Here's how the part is built. I have some questions about the finished solid (model axes, mm). Face numbers are marked on the shaded views. A direction names the side the tool comes from. Round coordinates to 2 decimals unless told otherwise and drop trailing zeros. Loops run counter-clockwise (first coordinate to the right, second up) from the corner with the lowest first, then second, coordinate; pieces in that order, holes last. Notation, with made-up numbers: M 28,65 L 68,65 A20 cw 68,92 Z; hole C 9,-16 d11. An arc over 180 degrees is marked long. Use a Markdown table: item, result.
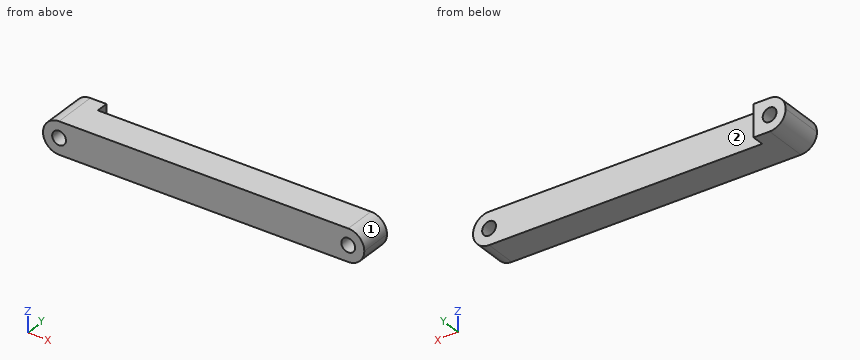
```python
from build123d import *

# Parameters (mm, degrees)
SKETCH_1_W          = 100
SKETCH_1_H          = 10
EXTRUDE_1_DEPTH     = 10
SKETCH_4_W          = 10
SKETCH_4_H          = 10
EXTRUDE_2_DEPTH     = 3.8
FILLET_1_R          = 5
SKETCH_2_R          = 2.15
CUT_EXTRUDE_1_DEPTH = 53.824615474


with BuildPart() as part:
    # 스케치1 → 보스-돌출1 (new body)
    with BuildSketch(Plane.XY):
        Rectangle(SKETCH_1_W, SKETCH_1_H)
    extrude(amount=EXTRUDE_1_DEPTH)

    # 스케치4 → 보스-돌출2 (add)
    with BuildSketch(Plane(origin=(0, 5, 0), x_dir=(1, 0, 0), z_dir=(0, 1, 0))):
        with Locations((-45, -5)):
            Rectangle(SKETCH_4_W, SKETCH_4_H)
    extrude(amount=EXTRUDE_2_DEPTH)

    # 필렛1
    fillet_1_edges = [part.edges().sort_by_distance(p)[0] for p in [
        (50, 0, 0),
        (50, 0, 10),
        (-50, 1.9, 0),
        (-50, 1.9, 10),
    ]]
    fillet(fillet_1_edges, radius=FILLET_1_R - 0.0001)  # a hair under: the kernel refuses the full size

    # 스케치2 → 컷-돌출1 (cut, through all)
    with BuildSketch(Plane(origin=(0, 8.8, 0), x_dir=(1, 0, 0), z_dir=(0, 1, 0))):
        with Locations(Location((-45, -5, 0), (0, 0, 270))):
            Circle(SKETCH_2_R)
        with Locations(Location((45, -5, 0), (0, 0, 270))):
            Circle(SKETCH_2_R)
    extrude(amount=-CUT_EXTRUDE_1_DEPTH, mode=Mode.SUBTRACT)


solid = part.part
```
Q1. For the marked faces 1 and 2, which set-ups out of +Z, -Z, +X, -X, +Y, -Y let a thin tool reach every point of the face, with its end or its side?
Return value:
| item | result |
|---|---|
| face 1 | +Z, +X, +Y, -Y |
| face 2 | +Z, -Z, +X, +Y |
Q2. Imagine slicing it at B-B, the plane z = 3.75. Please give me the cut outline in (x, y), then the cut area to 3 significant figures.
Return value:
| item | result |
|---|---|
| outline | M -49.84,-5 L -46.75,-5 L -46.75,8.8 L -49.84,8.8 Z; M -43.25,-5 L 43.25,-5 L 43.25,5 L -40,5 L -40,8.8 L -43.25,8.8 Z; M 46.75,-5 L 49.84,-5 L 49.84,5 L 46.75,5 Z |
| area | 951 mm^2 |
Q3. I need wall thicknesses on line 1 (X direction, y = 1.25, z = 5); line 2 (X direction, y = 4.25, z = 6); line 3 (Y direction, x = 8, z = 7). Which ranges of each line are inside material? Lowest first, please. Write a range as from..to.
Return value:
| item | result |
|---|---|
| line 1 | x = -50..-47.15, -42.85..42.85, 47.15..50 |
| line 2 | x = -49.9..-46.9, -43.1..43.1, 46.9..49.9 |
| line 3 | y = -5..5 |
Q4. Imagine slicing it at A-A, the plane y = -0.75. Give the number of separate pieces and of enclosed holes in the cut face, then the cut area to 3 significant figures.
Return value:
| item | result |
|---|---|
| separate pieces | 1 |
| enclosed holes | 2 |
| area | 949 mm^2 |
Q5. Imagine slicing it at D-D, the plane x = 9. Please give me the cut outline in (y, z), then the cut area to 3 significant figures.
Return value:
| item | result |
|---|---|
| outline | M -5,0 L 5,0 L 5,10 L -5,10 Z |
| area | 100 mm^2 |
Q6. Will these pins go through, and if not, where does the flat tip stop? P1, Ø1.5, axis at y = -0.5, z = 4.5, coming from the -X side; P2, Ø5, axis at x = 10, z = 6, coming from the +Y side; P3, Ø4, axis at x = 45, z = 5, coming from the +Y side; P4, Ø1.5, axis at y = -3.5, z = 2, coming from the +X side.
Return value:
| item | result |
|---|---|
| P1 | stops at x = -50 |
| P2 | stops at y = 5 |
| P3 | passes through |
| P4 | stops at x = 49.47 |
